from build123d import *

# Parameters (mm, degrees)
SKETCH1_W                       = 21
SKETCH1_H                       = 2.5
SKETCH1_H_2                     = 3
SKETCH1_W_2                     = 2
BOSS_EXTRUDE1_DEPTH             = 2
BOSS_EXTRUDE2_REACH             = 15.276
BOSS_EXTRUDE2_DIRECTION_2_REACH = 15.276
BOSS_EXTRUDE3_REACH             = 17.37
SKETCH5_R                       = 1.75
CUT_EXTRUDE1_DEPTH              = 14.720422734
SKETCH6_R                       = 3
CUT_EXTRUDE2_DEPTH              = 2
CHAMFER1_SIZE                   = 1


with BuildPart() as part:
    # Sketch1 → Boss-Extrude1 (new body)
    with BuildSketch(Plane(origin=(0, 0, 0), x_dir=(1, 0, 0), z_dir=(0, 1, 0))):
        with Locations((0, -2.75)):
            Rectangle(SKETCH1_W, SKETCH1_H)
        Rectangle(SKETCH1_W, SKETCH1_H_2)
        with Locations((-11.5, 0)):
            Rectangle(SKETCH1_W_2, SKETCH1_H_2)
        with Locations((11.5, 0)):
            Rectangle(SKETCH1_W_2, SKETCH1_H_2)
        with Locations((0, 2.75)):
            Rectangle(SKETCH1_W, SKETCH1_H)
    extrude(amount=BOSS_EXTRUDE1_DEPTH)

    # Boss-Extrude2: up to this face of the body (flat: up to its plane)
    boss_extrude2_end = Plane(part.part.faces().sort_by_distance((-11.5, 1, 1.5))[0])
    # Sketch3 → Boss-Extrude2 (add, up to the picked face)
    with BuildSketch(Plane.XY, mode=Mode.PRIVATE) as boss_extrude2_sk1:
        Polygon((-12.5, 2), (-3.5, 4), (3.5, 4), (12.5, 2), align=None)
    boss_extrude2_tool1 = split(extrude(boss_extrude2_sk1.sketch, amount=BOSS_EXTRUDE2_REACH, mode=Mode.PRIVATE), bisect_by=boss_extrude2_end, keep=Keep.BOTH, mode=Mode.PRIVATE)
    add(boss_extrude2_tool1.solids().sort_by(Axis((0, 2.8125, 0), (0, 0, 1)))[0])

    # Boss-Extrude2 direction 2: up to this face of the body (flat: up to its plane)
    boss_extrude2_direction_2_end = Plane(part.part.faces().sort_by_distance((-11.5, 1, -1.5))[0])
    # Sketch3 → Boss-Extrude2 direction 2 (add, up to the picked face)
    with BuildSketch(Plane.XY, mode=Mode.PRIVATE) as boss_extrude2_direction_2_sk1:
        Polygon((-12.5, 2), (-3.5, 4), (3.5, 4), (12.5, 2), align=None)
    boss_extrude2_direction_2_tool1 = split(extrude(boss_extrude2_direction_2_sk1.sketch, amount=-BOSS_EXTRUDE2_DIRECTION_2_REACH, mode=Mode.PRIVATE), bisect_by=boss_extrude2_direction_2_end, keep=Keep.BOTH, mode=Mode.PRIVATE)
    add(boss_extrude2_direction_2_tool1.solids().sort_by(Axis((0, 2.8125, 0), (0, 0, -1)))[0])

    # Boss-Extrude3: up to this face of the body (flat: up to its plane)
    boss_extrude3_end = Plane(part.part.faces().sort_by_distance((0, 1, -4))[0])
    # Sketch4 → Boss-Extrude3 (add, up to the picked face)
    with BuildSketch(Plane.XY.offset(4), mode=Mode.PRIVATE) as boss_extrude3_sk1:
        Polygon((10.5, 2), (3.5, 4), (-3.5, 4), (-10.5, 2), align=None)
    boss_extrude3_tool1 = split(extrude(boss_extrude3_sk1.sketch, amount=-BOSS_EXTRUDE3_REACH, mode=Mode.PRIVATE), bisect_by=boss_extrude3_end, keep=Keep.BOTH, mode=Mode.PRIVATE)
    add(boss_extrude3_tool1.solids().sort_by(Axis((0, 2.833333, 4), (0, 0, -1)))[0])

    # Sketch5 → Cut-Extrude1 (cut, through all)
    with BuildSketch(Plane(origin=(0, 4, 0), x_dir=(1, 0, 0), z_dir=(0, 1, 0))):
        with Locations(Location((0, 0, 0), (0, 0, 270))):
            Circle(SKETCH5_R)
    extrude(amount=-CUT_EXTRUDE1_DEPTH, mode=Mode.SUBTRACT)

    # Sketch6 → Cut-Extrude2 (cut)
    with BuildSketch(Plane(origin=(0, 4, 0), x_dir=(1, 0, 0), z_dir=(0, 1, 0))):
        with Locations(Location((0, 0, 0), (0, 0, 270))):
            Circle(SKETCH6_R)
    extrude(amount=-CUT_EXTRUDE2_DEPTH, mode=Mode.SUBTRACT)

    # Chamfer1
    chamfer1_edges = [part.edges().sort_by_distance(p)[0] for p in [
        (7, 3, 4),
        (0, 4, 4),
        (-7, 3, 4),
        (7, 3, -4),
        (0, 4, -4),
        (-7, 3, -4),
    ]]
    chamfer(chamfer1_edges, length=CHAMFER1_SIZE - 0.0001)  # a hair under: the kernel refuses the full size


solid = part.part
Geometry check sheet. Reference: the model listing, model coordinates, mm. A direction names the side the tool comes from. Give positions to 0.01 mm unless a question says otherwise; leave off trailing zeros. Write each loop counter-clockwise with the first axis right and the second up, starting at its lowest first coordinate (ties: lowest second). Pieces come first, ordered by that corner, then holes.
1) Set-up check for faces 5 (the face through (7, 3, 2)), 6 (the face through (-10.5, 1, -3)), 7 (the face through (-7, 3, -2)): record each of +Z, -Z, +X, -X, +Y, -Y from which the full face is reachable in a straight line by a thin tool's end or side.
Values follow:
face 5: +Z, +X, +Y
face 6: -Z, -X, +Y, -Y
face 7: -Z, -X, +Y
2) Cross-section at D-D (x = 9.5). Record the boundary of the cut face in (y, z), plus the area to 3 significant figures.
Values follow:
outline: (0, -4) - (1.25, -4) - (2.29, -3) - (2.29, -1.5) - (2.67, -1.5) - (2.67, 1.5) - (2.29, 1.5) - (2.29, 3) - (1.25, 4) - (0, 4) - close
area: 18.4 mm2
3) Cross-section at C-C (y = 0.6). Record the boundary of the cut face in (x, z), plus the area to 3 significant figures.
Values follow:
outline: (-12.5, -1.5) - (-10.5, -1.5) - (-10.5, -4) - (10.5, -4) - (10.5, -1.5) - (12.5, -1.5) - (12.5, 1.5) - (10.5, 1.5) - (10.5, 4) - (-10.5, 4) - (-10.5, 1.5) - (-12.5, 1.5) - close; hole circle Ø3.5 at (0, 0)
area: 170 mm2
4) Go/stop test with flat-tipped pins: pin 1 Ø2 at (y, z) = (1.5, 3.5) entering from +X; pin 2 Ø1.2 at (x, y) = (8, 2.5) entering from +Z; pin 3 Ø0.6 at (y, z) = (0.5, 3) entering from -X. Record where each tip stops, or that it passes through.
Values follow:
pin 1: stops at x = 10.5
pin 2: stops at z = 3.81
pin 3: stops at x = -10.5
5) Release check for a two-part mould opening along Z. For faces 1 (the face through (-1.71, 1.01, -0.38)), 2 (the face through (-7, 3, 2)), 3 (the face through (0, 3.5, 3.5)), 4 (the face through (-2, 2, 0)) record: released by +Z, released by -Z, zero draft, split by the parting line, or undercut.
Values follow:
face 1: undercut
face 2: zero draft
face 3: released by +Z
face 4: undercut
6) Cross-section at A-A (z = 0). Record the boundary of the cut face in (x, y), plus the area to 3 significant figures.
Values follow:
outline: (-12.5, 0) - (-1.75, 0) - (-1.75, 2) - (-3, 2) - (-3, 4) - (-3.5, 4) - (-12.5, 2) - close; (1.75, 0) - (12.5, 0) - (12.5, 2) - (3.5, 4) - (3, 4) - (3, 2) - (1.75, 2) - close
area: 63.0 mm2
7) Thickness scan on line 1 (X direction, y = 1.45, z = -2.75); line 2 (Z direction, x = 11, y = 0.45); line 3 (Y direction, x = -8, z = 1). Record the ranges inside material, lowest first.
Values follow:
line 1: x = -10.5 to 10.5
line 2: z = -1.5 to 1.5
line 3: y = 0 to 3
